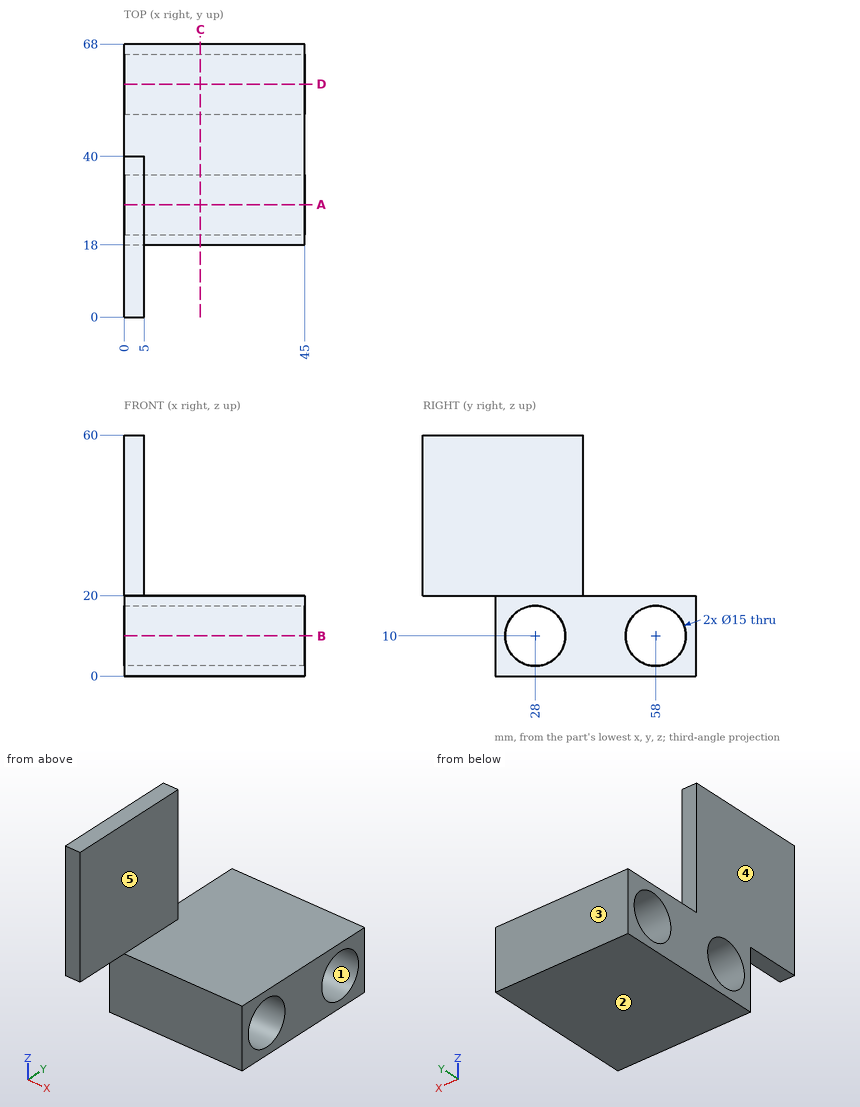
Here's the drawing with two shaded views (mm, measured from the low corner). I have some questions. A direction names the side the tool comes from. Coordinates: 2 decimals unless noted, no trailing zeros. Write each loop counter-clockwise with the first axis right and the second up, starting at its lowest first coordinate (ties: lowest second). Pieces come first, ordered by that corner, then holes. Notation, with made-up numbers: M 50,-18 L 69,-18 A9 ccw 69,-7 Z; hole C -19.5,9.25 d3. An arc over 180 degrees is marked long. Answer as CSV lines item,"result".
Item 1: We'd pull the mould along Y, two halves only. Please class the marked faces 1, 2 and 3: +Y half, -Y half, draft (parallel to the pull), parting line (faces both ways), or undercut.
Geometry results:
face 1,"undercut"
face 2,"draft"
face 3,"+Y half"
Item 2: Please list where these lines run through material, in increasing order: line 1 along Y through (x, z) = (12, 10); line 2 along Y through (x, z) = (41.5, 3.5); line 3 along Z through (x, y) = (41, 40).
Geometry results:
line 1,"y = 18 to 20.5, 35.5 to 50.5, 65.5 to 68"
line 2,"y = 18 to 24.26, 31.74 to 54.26, 61.74 to 68"
line 3,"z = 0 to 20"
Item 3: Imagine slicing it at B-B on z = 10. List the corners of the cut face in (x, y) for me.
Geometry results:
outline,"M 0,18 L 45,18 L 45,20.5 L 0,20.5 Z; M 0,35.5 L 45,35.5 L 45,50.5 L 0,50.5 Z; M 0,65.5 L 45,65.5 L 45,68 L 0,68 Z"
Item 4: Imagine slicing it at A-A on y = 28. List the corners of the cut face in (x, z) for me.
Geometry results:
outline,"M 0,0 L 45,0 L 45,2.5 L 0,2.5 Z; M 0,17.5 L 45,17.5 L 45,20 L 5,20 L 5,60 L 0,60 Z"
Item 5: Imagine slicing it at C-C on x = 19. List the corners of the cut face in (y, z) for me, plus the area to 3 significant figures.
Geometry results:
outline,"M 18,0 L 68,0 L 68,20 L 18,20 Z; hole C 28,10 d15; hole C 58,10 d15"
area,"647 mm2"
Item 6: On a 3-axis mill with a long thin cutter (end or side, diameter ignored), from which of +Z, -Z, +X, -X, +Y, -Y can I reach the whole of each face in a straight line? I mean the marked faces 4 and 5. Say none if no direction works.
Geometry results:
face 4,"+Z, -Z, -X, +Y, -Y"
face 5,"+Z, +X, +Y, -Y"
Item 7: Imagine slicing it at D-D on y = 58. List the corners of the cut face in (x, z) for me.
Geometry results:
outline,"M 0,0 L 45,0 L 45,2.5 L 0,2.5 Z; M 0,17.5 L 45,17.5 L 45,20 L 0,20 Z"
Item 8: I'm going to push flat-ended pins straight in: P1, Ø8, axis at x = 6, z = 11.5, coming from the -Y side; P2, Ø4, axis at x = 2.5, z = 47.5, coming from the +Y side; P3, Ø1.5, axis at x = 3.5, y = 5, coming from the -Z side. Where does each tip first touch, or does it pass through?
Geometry results:
P1,"stops at y = 18"
P2,"stops at y = 40"
P3,"stops at z = 20"
